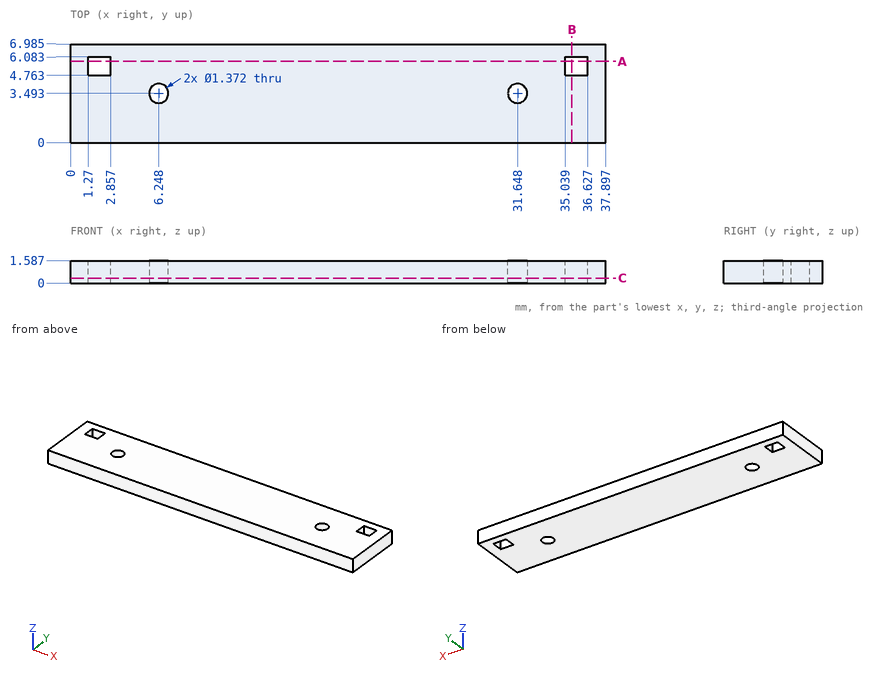
Here's the drawing with two shaded views (mm, measured from the low corner). I have some questions. Coordinates: 2 decimals unless noted, no trailing zeros. Order: outer loops, then holes, each group sorted by start corner. A loop starts at its lowest first (then second) coordinate and runs counter-clockwise, first axis right, second up.
Item 1: I'm going to push a flat-ended pin straight in: pin 1 Ø0.8 at (x, y) = (31.65, 3.49) entering from +Z. Where does the tip first touch, or does it pass through?
Response values:
pin 1: passes through
Item 2: If we section it at A-A, the plane y = 5.75: List the corners of the cut face in (x, z) for me.
Response values:
outline: (0, 0) - (1.27, 0) - (1.27, 1.59) - (0, 1.59) - close; (2.86, 0) - (35.04, 0) - (35.04, 1.59) - (2.86, 1.59) - close; (36.63, 0) - (37.9, 0) - (37.9, 1.59) - (36.63, 1.59) - close
Item 3: If we section it at B-B, the plane x = 35.5: List the corners of the cut face in (y, z) for me (1 decimal).
Response values:
outline: (0, 0) - (4.8, 0) - (4.8, 1.6) - (0, 1.6) - close; (6.1, 0) - (7, 0) - (7, 1.6) - (6.1, 1.6) - close
Item 4: I need wall thicknesses on probe 1 along X at (y, z) = (5.25, 1.2); probe 2 along X at (y, z) = (4, 0.2) (1 decimal); probe 3 along Y at (x, z) = (2, 1.05) (1 decimal). Which ranges of each line are inside material? Lowest first, please.
Response values:
probe 1: x = 0 to 1.27, 2.86 to 35.04, 36.63 to 37.9
probe 2: x = 0 to 5.8, 6.7 to 31.2, 32.1 to 37.9
probe 3: y = 0 to 4.8, 6.1 to 7
Item 5: If we section it at C-C, the plane z = 0.35: List the corners of the cut face in (x, y) for me (1 decimal).
Response values:
outline: (0, 0) - (37.9, 0) - (37.9, 7) - (0, 7) - close; hole (1.3, 4.8) - (2.9, 4.8) - (2.9, 6.1) - (1.3, 6.1) - close; hole circle Ø1.4 at (6.2, 3.5); hole circle Ø1.4 at (31.6, 3.5); hole (35, 4.8) - (36.6, 4.8) - (36.6, 6.1) - (35, 6.1) - close
